```python
from build123d import *

# Parameters (mm, degrees)
F0_R     = 12.5
F0_R_2   = 5
F1_DEPTH = 15
F2_DEPTH = 15
F0_R_3   = 2.75
F3_DEPTH = 5
F4_DEPTH = 3
F5_DEPTH = 3
F7_R     = 0.5
F8_DEPTH = 15


# Not quite as in the source:
# - a fillet or chamfer that OpenCascade refuses, or shapes differently, is made with other operations: its cross-section is extruded or revolved along the edge and cut away or added


with BuildPart() as f1:
    # F0 (on Front) → F1 (new body)
    with BuildSketch(Plane.XZ):
        Circle(F0_R)
        Circle(F0_R_2, mode=Mode.SUBTRACT)
    extrude(amount=F1_DEPTH)

    # F0 (on Front) → F2 (join)
    with BuildSketch(Plane.XZ):
        Circle(F0_R_2)
        Polygon((-4.2491954474, -2.4551316428), (-4.250804096, 2.4523453817), (-0.0016086486, 4.9074770245), (4.2491954474, 2.4551316428), (4.250804096, -2.4523453817), (0.0016086486, -4.9074770245), align=None, mode=Mode.SUBTRACT)
    extrude(amount=F2_DEPTH)

    # F0 (on Front) → F3 (join)
    with BuildSketch(Plane.XZ):
        Polygon((-0.0016086486, 4.9074770245), (-4.250804096, 2.4523453817), (-4.2491954474, -2.4551316428), (0.0016086486, -4.9074770245), (4.250804096, -2.4523453817), (4.2491954474, 2.4551316428), align=None)
        Circle(F0_R_3, mode=Mode.SUBTRACT)
    extrude(amount=F3_DEPTH)

    # F0 (on Front) → F4 (join)
    with BuildSketch(Plane.XZ):
        Circle(F0_R_2)
        Polygon((-4.2491954474, -2.4551316428), (-4.250804096, 2.4523453817), (-0.0016086486, 4.9074770245), (4.2491954474, 2.4551316428), (4.250804096, -2.4523453817), (0.0016086486, -4.9074770245), align=None, mode=Mode.SUBTRACT)
    extrude(amount=-F4_DEPTH)

    # F0 (on Front) → F5 (join)
    with BuildSketch(Plane.XZ):
        Polygon((-0.0016086486, 4.9074770245), (-4.250804096, 2.4523453817), (-4.2491954474, -2.4551316428), (0.0016086486, -4.9074770245), (4.250804096, -2.4523453817), (4.2491954474, 2.4551316428), align=None)
        Circle(F0_R_3, mode=Mode.SUBTRACT)
    extrude(amount=-F5_DEPTH)

    # F6: chamfer of 2.5 on 1 edges, made by hand

    # F6_s1 → F6_t2 (revolve, cut)
    with BuildSketch(Plane.XY):
        Polygon((2.5, 3), (5, 0.5), (5, 3), align=None)
    revolve(axis=Axis((0, 3, 0), (0, -1, 0)), mode=Mode.SUBTRACT)

    # F7 (on Front) → F8 (cut)
    with BuildSketch(Plane.XZ):
        with Locations((-5.3183648548, -11.3121613881)):
            Circle(F7_R)
        with Locations((-3.6922583147, -11.94224554)):
            Circle(F7_R)
        with Locations((-1.9942861663, -12.3398874665)):
            Circle(F7_R)
        with Locations((-0.2574975062, -12.4973475199)):
            Circle(F7_R)
        with Locations((1.4843030499, -12.4115609194)):
            Circle(F7_R)
        with Locations((3.1972133356, -12.0841974035)):
            Circle(F7_R)
        with Locations((4.8478935004, -11.5216287307)):
            Circle(F7_R)
        with Locations((6.4042149327, -10.7348046603)):
            Circle(F7_R)
        with Locations((7.835885606, -9.7390398279)):
            Circle(F7_R)
        with Locations((9.1150396792, -8.5537156632)):
            Circle(F7_R)
        with Locations((10.2167798732, -7.2019031529)):
            Circle(F7_R)
        with Locations((11.1196620684, -5.7099137897)):
            Circle(F7_R)
        with Locations((11.8061126898, -4.1067874495)):
            Circle(F7_R)
        with Locations((12.262770757, -2.423727163)):
            Circle(F7_R)
        with Locations((12.4807479401, -0.6934917843)):
            Circle(F7_R)
        with Locations((12.4558015612, 1.0502416232)):
            Circle(F7_R)
        with Locations((12.1884171732, 2.7735332722)):
            Circle(F7_R)
        with Locations((11.683799109, 4.4428412508)):
            Circle(F7_R)
        with Locations((10.9517691853, 6.0256743782)):
            Circle(F7_R)
        with Locations((10.0065755319, 7.4912246078)):
            Circle(F7_R)
        with Locations((8.866615268, 8.8109666717)):
            Circle(F7_R)
        with Locations((7.5540764236, 9.9592132916)):
            Circle(F7_R)
        with Locations((6.0945060742, 10.9136151532)):
            Circle(F7_R)
        with Locations((4.5163130964, 11.6555959099)):
            Circle(F7_R)
        with Locations((2.8502152215, 12.1707137503)):
            Circle(F7_R)
        with Locations((1.1286411494, 12.4489424915)):
            Circle(F7_R)
        with Locations((-0.6149006389, 12.4848667275)):
            Circle(F7_R)
        with Locations((-2.3464740857, 12.2777872341)):
            Circle(F7_R)
        with Locations((-4.0323760835, 11.8317345779)):
            Circle(F7_R)
        with Locations((-5.6397924676, 11.1553906665)):
            Circle(F7_R)
        with Locations((-7.1374367064, 10.2619197649)):
            Circle(F7_R)
        with Locations((-8.4961588585, 9.1687122678)):
            Circle(F7_R)
        with Locations((-9.6895129427, 7.8970462157)):
            Circle(F7_R)
        with Locations((-10.6942716791, 6.4716731418)):
            Circle(F7_R)
        with Locations((-11.4908785818, 4.9203363116)):
            Circle(F7_R)
        with Locations((-12.0638286036, 3.2732307318)):
            Circle(F7_R)
        with Locations((-12.401969924, 1.5624154391)):
            Circle(F7_R)
        with Locations((-12.4987210069, -0.1788104928)):
            Circle(F7_R)
        with Locations((-12.3521987024, -1.916556082)):
            Circle(F7_R)
        with Locations((-11.9652549007, -3.616998087)):
            Circle(F7_R)
        with Locations((-11.3454210226, -5.2470393386)):
            Circle(F7_R)
        with Locations((-10.5047614295, -6.7749529378)):
            Circle(F7_R)
        with Locations((-9.4596386041, -8.1709997846)):
            Circle(F7_R)
        with Locations((-8.2303946735, -9.4080074148)):
            Circle(F7_R)
        with Locations((-6.8409554726, -10.4618988822)):
            Circle(F7_R)
    extrude(amount=F8_DEPTH, mode=Mode.SUBTRACT)


solid = f1.part
```
Design review of the part built by this model. Coordinates are the model's own, in mm. A direction names the side the tool comes from. Give positions to 0.01 mm unless a question says otherwise; leave off trailing zeros. One line per item, written item: value.
Q1. For pin 1 Ø1.5 at (y, z) = (-11.5, -1) entering from +X; pin 2 Ø2 at (y, z) = (-12.5, 1.5) entering from +X; pin 3 Ø1 at (y, z) = (-0.5, -8.5) entering from -X; pin 4 Ø5 at (x, z) = (0, 0) entering from -Y, all flat-tipped, find the tip position at first contact; note any pin that passes through.
Numbers:
pin 1: stops at x = 12.44
pin 2: stops at x = 12.49
pin 3: stops at x = -9.13
pin 4: passes through
Q2. Draft analysis for pull direction X (two halves, no side actions). For faces 3 (the cylindrical face through (10.51, -7.4, 5.79)), 4 (the cylindrical face through (-1.08, 0.25, -4.88)), 5 (the flat face through (-3, -5, 0)), state which applies: pulls with the +X half, pulls with the -X half, needs draft (parallel to the pull), parting line crosses it, or undercut.
Numbers:
face 3: undercut
face 4: parting line crosses it
face 5: undercut
Q3. Machinability: for faces 1 (the cylindrical face through (6.16, -7.4, -10.3)), 2 (the flat face through (-2.09, -9.93, -3.7)), which of the approach directions +Z, -Z, +X, -X, +Y, -Y give a long, thin tool a straight path to every point of the face, cutting with its end or side? Answer none if there is none.
Numbers:
face 1: +Y, -Y
face 2: -Y
Q4. For L1, parallel to Z at x = 3.25, y = -8.25; L2, parallel to Y at x = 6.5, z = 1.5; L3, parallel to Z at x = 0, y = -2.2, list the stretches that pass through material, from the lowest coordinate up.
Numbers:
L1: z = -11.59 to -3.03, 3.03 to 11.87
L2: y = -15 to 0
L3: z = -12.07 to -2.75, 2.75 to 12.5
